Here's the drawing with two shaded views (mm, measured from the low corner). I have some questions. A direction names the side the tool comes from. Coordinates: 2 decimals unless noted, no trailing zeros. Write each loop counter-clockwise with the first axis right and the second up, starting at its lowest first coordinate (ties: lowest second). Pieces come first, ordered by that corner, then holes.
Item 1: If we section it at C-C (x = 8.5): Please give me the cut outline in (y, z).
Item 2: If we section it at B-B (y = 8): Please give me the cut outline in (x, z).
Item 3: If I drill on line 1 (Z direction, x = 7.75, y = 9.75); line 2 (Y direction, x = 23.5, z = 3.75); line 3 (X direction, y = 5.5, z = 3.75), over which ranges is the centre line in solid material (lowest first)?
Item 4: If we section it at A-A (z = 4): Please give me the cut outline in (x, y), then the cut area to 3 significant figures.
Item 5: If we section it at D-D (z = 2): Please give me the cut outline in (x, y).
Item 6: For the marked faces 1, 2 and 3, which set-ups out of +Z, -Z, +X, -X, +Y, -Y let a thin tool reach every point of the face, with its end or its side?
Item 7: I'm going to push flat-ended pins straight in: pin 1 Ø0.8 at (y, z) = (1.5, 4) entering from +X; pin 2 Ø4 at (x, y) = (15.5, 3.5) entering from -Z; pin 3 Ø1.5 at (y, z) = (5.5, 2.5) entering from -X. Where does each tip first touch, or does it pass through?
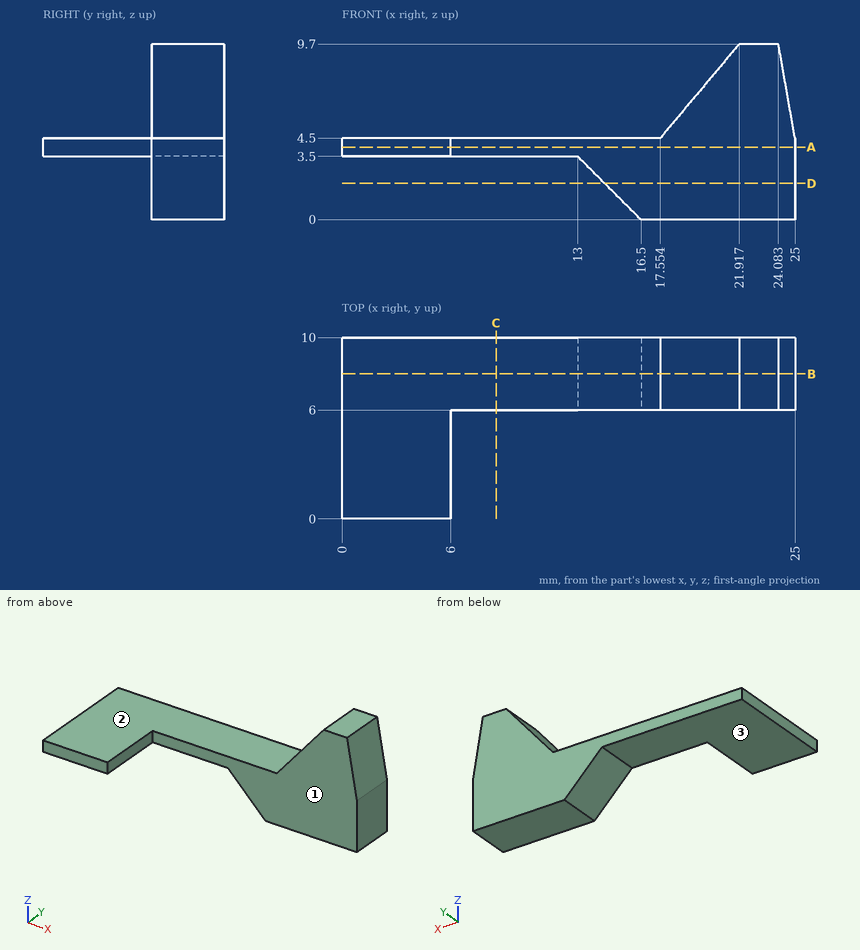
Answer list:
1. outline: (6, 3.5) - (10, 3.5) - (10, 4.5) - (6, 4.5) - close
2. outline: (0, 3.5) - (13, 3.5) - (16.5, 0) - (25, 0) - (25, 4.5) - (24.08, 9.7) - (21.92, 9.7) - (17.55, 4.5) - (0, 4.5) - close
3. line 1: z = 3.5 to 4.5
3. line 2: y = 6 to 10
3. line 3: x = 0 to 6
4. outline: (0, 0) - (6, 0) - (6, 6) - (25, 6) - (25, 10) - (0, 10) - close
4. area: 136 mm2
5. outline: (14.5, 6) - (25, 6) - (25, 10) - (14.5, 10) - close
6. face 1: +Z, -Z, +X, -Y
6. face 2: +Z, -X, +Y, -Y
6. face 3: -Z, -X, +Y, -Y
7. pin 1: stops at x = 6
7. pin 2: passes through
7. pin 3: stops at x = 13.44
